Verification items for the finished model (mm, model axes). Face numbers are marked on the shaded views. A direction names the side the tool comes from. Give positions to 0.01 mm unless a question says otherwise; leave off trailing zeros. Order: outer loops, then holes, each group sorted by start corner. A loop starts at its lowest first (then second) coordinate and runs counter-clockwise, first axis right, second up.
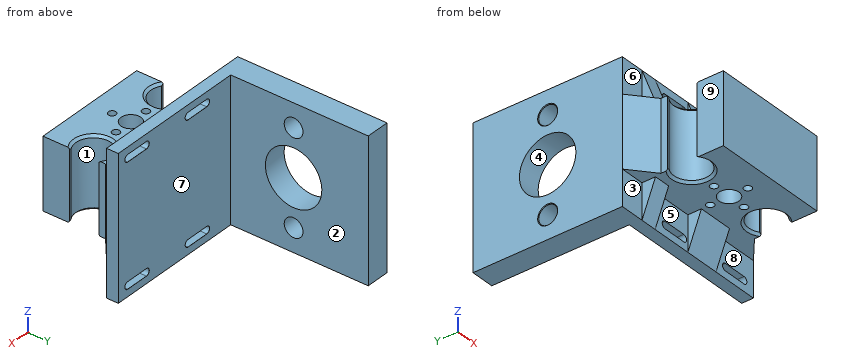
from build123d import *

# Parameters (mm, degrees)
SKETCH_1_W               = 50
SKETCH_1_H               = 35
EXTRUDE_1_DEPTH          = 30
HOLE_WIZARD_362_D        = 8.5
HOLE_WIZARD_467_D        = 3.2
HOLE_WIZARD_621_D        = 15
CHAMFER_1_SIZE           = 1
CHAMFER_1_SIZE_2         = 0.708203932
SKETCH_8_W               = 70
SKETCH_8_H               = 60
SKETCH_8_W_2             = 50
SKETCH_8_H_2             = 30
EXTRUDE_2_DEPTH          = 63.5
HOLE_WIZARD_1_D          = 24
HOLE_WIZARD_2_D          = 8
CHAMFER_2_SIZE           = 0.25
CUT_EXTRUDE_2_DEPTH      = 107.705201373
CUT_EXTRUDE_2_DEPTH_BACK = 107.705201373
SKETCH_14_W              = 60
SKETCH_14_H              = 58.5
MM_START                 = 17
MM_2_DEPTH               = 5.5
RIB_1_REACH              = 95.199
SKETCH_25_WALL_W         = 201.46144539
SKETCH_25_WALL_H         = 30
RIB_2_REACH              = 101.05
SKETCH_26_WALL_W         = 216.17250262
SKETCH_26_WALL_H         = 15
RIB_4_REACH              = 108.5
SKETCH_27_WALL_W         = 231.071518272
SKETCH_27_WALL_H         = 7


with BuildPart() as part:
    # 草图1 → 凸台-拉伸1 (new body)
    with BuildSketch(Plane.XY):
        Rectangle(SKETCH_1_W, SKETCH_1_H)
    extrude(amount=EXTRUDE_1_DEPTH)

    # Hole Wizard 362 (through all)
    with Locations(Plane.XY.offset(30)):
        with Locations((0, 0)):
            Hole(HOLE_WIZARD_362_D / 2)

    # Hole Wizard 467 (through all)
    with Locations(Plane.XY.offset(30)):
        with Locations((8, 0), (0, 8), (-8, 0), (0, -8)):
            Hole(HOLE_WIZARD_467_D / 2)

    # Hole Wizard 621 (through all)
    with Locations(Plane.XY.offset(30)):
        with Locations((20, 0), (-20, 0)):
            Hole(HOLE_WIZARD_621_D / 2)

    # 倒角1
    # the kernel refuses this chamfer: 1, 0.708203932 mm, written as the material it takes off along each edge
    with BuildSketch(Plane(origin=(-20, 0, 0), x_dir=(-0.8790200859122482, 0.4767847402789059, 0), z_dir=(-0.4767847402789059, -0.8790200859122482, 0))) as chamfer_1_piece_1:
        Polygon((7.5, -CHAMFER_1_SIZE), (7.5 + CHAMFER_1_SIZE, 0), (7.5, 0), align=None)
    revolve(axis=Axis((-20, 0, 0), (0, 0, -1)), revolution_arc=303.048763938, mode=Mode.SUBTRACT)
    with BuildSketch(Plane(origin=(-20, 0, 30), x_dir=(-0.879020085912248, 0.47678474027890627, 0), z_dir=(-0.47678474027890627, -0.879020085912248, 0))) as chamfer_1_piece_2:
        Polygon((7.5 + CHAMFER_1_SIZE, 0), (7.5, CHAMFER_1_SIZE), (7.5, 0), align=None)
    revolve(axis=Axis((-20, 0, 30), (0, 0, -1)), revolution_arc=303.048763938, mode=Mode.SUBTRACT)
    with BuildSketch(Plane(origin=(20, 0, 30), x_dir=(0.879020085912248, -0.4767847402789061, 0), z_dir=(0.4767847402789061, 0.879020085912248, 0))) as chamfer_1_piece_3:
        Polygon((7.5 + CHAMFER_1_SIZE, 0), (7.5, CHAMFER_1_SIZE), (7.5, 0), align=None)
    revolve(axis=Axis((20, 0, 30), (0, 0, -1)), revolution_arc=303.048763938, mode=Mode.SUBTRACT)
    with BuildSketch(Plane(origin=(20, 0, 0), x_dir=(0.8790200859122481, 0.476784740278906, 0), z_dir=(0.476784740278906, -0.8790200859122481, 0))) as chamfer_1_piece_4:
        Polygon((7.5, CHAMFER_1_SIZE), (7.5 + CHAMFER_1_SIZE, 0), (7.5, 0), align=None)
    revolve(axis=Axis((20, 0, 0), (0, 0, 1)), revolution_arc=303.048763938, mode=Mode.SUBTRACT)
    with BuildSketch(Plane(origin=(-25, 5.590169944, 32.778051389), x_dir=(0.7914486393779661, 0.611235675682274, 0), z_dir=(0, 0, -1)), Plane(origin=(25, -5.590169944, 32.778051389), x_dir=(-0.7914486393779661, -0.611235675682274, 0), z_dir=(0, 0, -1))) as chamfer_1_piece_5:
        with BuildLine():
            Line((1.080663788, 0), (CHAMFER_1_SIZE_2 * 0.611235676113, -CHAMFER_1_SIZE_2 * 0.791448639936))
            Line((CHAMFER_1_SIZE_2 * 0.611235676113, -CHAMFER_1_SIZE_2 * 0.791448639936), (0, 0))
            ThreePointArc((0, 0), (0.555522087, -0.019473843), (1.080663788, 0))
        make_face()
    extrude(amount=35.556102778, mode=Mode.SUBTRACT)
    with BuildSketch(Plane(origin=(-25, -5.590169944, 32.778051389), x_dir=(0.7914486393779665, -0.6112356756822735, 0), z_dir=(0, 0, -1))) as chamfer_1_piece_6:
        with BuildLine():
            Line((1.080663788, 0), (CHAMFER_1_SIZE_2 * 0.611235676113, CHAMFER_1_SIZE_2 * 0.791448639936))
            Line((CHAMFER_1_SIZE_2 * 0.611235676113, CHAMFER_1_SIZE_2 * 0.791448639936), (0, 0))
            ThreePointArc((0, 0), (0.555522087, 0.019473843), (1.080663788, 0))
        make_face()
    extrude(amount=35.556102778, mode=Mode.SUBTRACT)
    with BuildSketch(Plane(origin=(25, 5.590169944, 32.778051389), x_dir=(0, 1, 0), z_dir=(0, 0, -1))) as chamfer_1_piece_7:
        with BuildLine():
            Line((CHAMFER_1_SIZE_2, 0), (0.660540261, -0.855289885))
            ThreePointArc((0.660540261, -0.855289885), (0.354967464, -0.427764092), (0, 0))
            Line((0, 0), (CHAMFER_1_SIZE_2, 0))
        make_face()
    extrude(amount=35.556102778, mode=Mode.SUBTRACT)

    # 草图8 → 凸台-拉伸2 (add)
    # profile 1 of 5: a face of its own
    with BuildSketch(Plane(origin=(0, 17.5, 0), x_dir=(1, 0, 0), z_dir=(0, 1, 0))):
        with Locations((0, -15)):
            Rectangle(SKETCH_8_W, SKETCH_8_H)
        with Locations((0, -15)):
            Rectangle(SKETCH_8_W_2, SKETCH_8_H_2, mode=Mode.SUBTRACT)
    # profile 2 of 5: a face of its own
    with BuildSketch(Plane(origin=(0, 17.5, 0), x_dir=(1, 0, 0), z_dir=(0, 1, 0))):
        Polygon((25, 0), (0, -15), (25, -30), align=None)
    # profile 3 of 5: a face of its own
    with BuildSketch(Plane(origin=(0, 17.5, 0), x_dir=(1, 0, 0), z_dir=(0, 1, 0))):
        Polygon((25, -30), (0, -15), (-25, -30), align=None)
    # profile 4 of 5: a face of its own
    with BuildSketch(Plane(origin=(0, 17.5, 0), x_dir=(1, 0, 0), z_dir=(0, 1, 0))):
        Polygon((0, -15), (-25, 0), (-25, -30), align=None)
    # profile 5 of 5: a face of its own
    with BuildSketch(Plane(origin=(0, 17.5, 0), x_dir=(1, 0, 0), z_dir=(0, 1, 0))):
        Polygon((25, 0), (-25, 0), (0, -15), align=None)
    extrude(amount=EXTRUDE_2_DEPTH)

    # 孔1 (through all)
    with Locations(Plane(origin=(35, 0, 0), x_dir=(0, 0, -1), z_dir=(1, 0, 0))):
        with Locations((-15, 49.25)):
            Hole(HOLE_WIZARD_1_D / 2)

    # 孔2 (through all)
    with Locations(Plane(origin=(35, 0, 0), x_dir=(0, 0, -1), z_dir=(1, 0, 0))):
        with Locations((5, 49.25), (-35, 49.25)):
            Hole(HOLE_WIZARD_2_D / 2)

    # 倒角2
    chamfer_2_edges = [part.edges().sort_by_distance(p)[0] for p in [
        (-35, 49.25, 31),
        (-35, 49.25, -9),
    ]]
    chamfer(chamfer_2_edges, length=CHAMFER_2_SIZE)

    # 草图14 → 切除-拉伸2 (cut, two sides: drawn at the far end of the back side and taken through both)
    with BuildSketch(Plane.XY.offset(45).offset(-CUT_EXTRUDE_2_DEPTH_BACK)):
        with Locations((5, 51.75)):
            Rectangle(SKETCH_14_W, SKETCH_14_H)
    extrude(amount=CUT_EXTRUDE_2_DEPTH + CUT_EXTRUDE_2_DEPTH_BACK, mode=Mode.SUBTRACT)

    # 大小mm 暗销槽口2: read off the stored shape, not the designer's step
    # 大小mm 暗销槽口2 outline → 大小mm 暗销槽口2 (cut)
    with BuildSketch(Plane(origin=(0, 0, 0), x_dir=(1, 0, 0), z_dir=(0, 1, 0)).offset(MM_START)):
        with BuildLine():
            Line((30, 11.959259259), (20, 11.959259259))
            ThreePointArc((20, 11.959259259), (18.5, 10.459259259), (20, 8.959259259))
            Line((20, 8.959259259), (30, 8.959259259))
            ThreePointArc((30, 8.959259259), (31.5, 10.459259259), (30, 11.959259259))
        make_face()
        with BuildLine():
            ThreePointArc((-12.203065134, 11.959259259), (-13.703065134, 10.459259259), (-12.203065134, 8.959259259))
            Line((-12.203065134, 8.959259259), (-2.203065134, 8.959259259))
            ThreePointArc((-2.203065134, 8.959259259), (-0.703065134, 10.459259259), (-2.203065134, 11.959259259))
            Line((-2.203065134, 11.959259259), (-12.203065134, 11.959259259))
        make_face()
    mm_2 = extrude(amount=MM_2_DEPTH, mode=Mode.SUBTRACT)

    # mm _2 2: loft between two sections, ruled curve by curve
    mm_2_2_from = [
        Edge.make_three_point_arc((30, 22.475, -8.959259259), (31.060660172, 22.475, -9.398599087), (31.5, 22.475, -10.459259259)),
        Edge.make_three_point_arc((31.5, 22.475, -10.459259259), (31.060660172, 22.475, -11.519919431), (30, 22.475, -11.959259259)),
        Edge.make_three_point_arc((20, 22.475, -11.959259259), (18.939339828, 22.475, -11.519919431), (18.5, 22.475, -10.459259259)),
        Edge.make_three_point_arc((18.5, 22.475, -10.459259259), (18.939339828, 22.475, -9.398599087), (20, 22.475, -8.959259259)),
        Edge.make_line((30, 22.475, -11.959259259), (20, 22.475, -11.959259259)),
        Edge.make_line((30, 22.475, -8.959259259), (20, 22.475, -8.959259259)),
    ]
    mm_2_2_to = [
        Edge.make_three_point_arc((30, 22.5, -8.934259259), (31.078337841, 22.5, -9.380921418), (31.525, 22.5, -10.459259259)),
        Edge.make_three_point_arc((31.525, 22.5, -10.459259259), (31.078337841, 22.5, -11.537597101), (30, 22.5, -11.984259259)),
        Edge.make_three_point_arc((20, 22.5, -11.984259259), (18.921662159, 22.5, -11.537597101), (18.475, 22.5, -10.459259259)),
        Edge.make_three_point_arc((18.475, 22.5, -10.459259259), (18.921662159, 22.5, -9.380921418), (20, 22.5, -8.934259259)),
        Edge.make_line((30, 22.5, -11.984259259), (20, 22.5, -11.984259259)),
        Edge.make_line((30, 22.5, -8.934259259), (20, 22.5, -8.934259259)),
    ]
    mm_2_2 = Solid(Shell([*[Face.make_surface_from_curves(mm_2_2_from[k], mm_2_2_to[k]) for k in range(6)], Face(Wire(mm_2_2_from)), Face(Wire(mm_2_2_to))]))
    add(mm_2_2, mode=Mode.SUBTRACT)

    # mm _2 3: loft between two sections, ruled curve by curve
    mm_2_3_from = [
        Edge.make_three_point_arc((-2.203065134, 22.475, -8.959259259), (-1.142404962, 22.475, -9.398599087), (-0.703065134, 22.475, -10.459259259)),
        Edge.make_three_point_arc((-0.703065134, 22.475, -10.459259259), (-1.142404962, 22.475, -11.519919431), (-2.203065134, 22.475, -11.959259259)),
        Edge.make_three_point_arc((-12.203065134, 22.475, -11.959259259), (-13.263725306, 22.475, -11.519919431), (-13.703065134, 22.475, -10.459259259)),
        Edge.make_three_point_arc((-13.703065134, 22.475, -10.459259259), (-13.263725306, 22.475, -9.398599087), (-12.203065134, 22.475, -8.959259259)),
        Edge.make_line((-2.203065134, 22.475, -11.959259259), (-12.203065134, 22.475, -11.959259259)),
        Edge.make_line((-2.203065134, 22.475, -8.959259259), (-12.203065134, 22.475, -8.959259259)),
    ]
    mm_2_3_to = [
        Edge.make_three_point_arc((-2.203065134, 22.5, -8.934259259), (-1.124727293, 22.5, -9.380921418), (-0.678065134, 22.5, -10.459259259)),
        Edge.make_three_point_arc((-0.678065134, 22.5, -10.459259259), (-1.124727293, 22.5, -11.537597101), (-2.203065134, 22.5, -11.984259259)),
        Edge.make_three_point_arc((-12.203065134, 22.5, -11.984259259), (-13.281402975, 22.5, -11.537597101), (-13.728065134, 22.5, -10.459259259)),
        Edge.make_three_point_arc((-13.728065134, 22.5, -10.459259259), (-13.281402975, 22.5, -9.380921418), (-12.203065134, 22.5, -8.934259259)),
        Edge.make_line((-2.203065134, 22.5, -11.984259259), (-12.203065134, 22.5, -11.984259259)),
        Edge.make_line((-2.203065134, 22.5, -8.934259259), (-12.203065134, 22.5, -8.934259259)),
    ]
    mm_2_3 = Solid(Shell([*[Face.make_surface_from_curves(mm_2_3_from[k], mm_2_3_to[k]) for k in range(6)], Face(Wire(mm_2_3_from)), Face(Wire(mm_2_3_to))]))
    add(mm_2_3, mode=Mode.SUBTRACT)

    # 镜向1: 大小mm 暗销槽口2, mm _2 2, mm _2 3 across plane
    add(mm_2.mirror(Plane(origin=(0, 0, 15), x_dir=(1, 0, 0), z_dir=(0, 0, -1))), mode=Mode.SUBTRACT)
    add(mm_2_2.mirror(Plane(origin=(0, 0, 15), x_dir=(1, 0, 0), z_dir=(0, 0, -1))), mode=Mode.SUBTRACT)
    add(mm_2_3.mirror(Plane(origin=(0, 0, 15), x_dir=(1, 0, 0), z_dir=(0, 0, -1))), mode=Mode.SUBTRACT)

    # 草图25 wall → 筋1 (add, up to next)
    with BuildSketch(Plane(origin=(-30, 13.296768148, 15), x_dir=(-0.765461137236, 0.6434821267, 0), z_dir=(0.6434821267, 0.765461137236, 0)), mode=Mode.PRIVATE) as rib_1_sk1:
        Rectangle(SKETCH_25_WALL_W, SKETCH_25_WALL_H)
    rib_1_tool1 = extrude(rib_1_sk1.sketch, amount=RIB_1_REACH, mode=Mode.PRIVATE) - part.part
    rib_1 = rib_1_tool1.solids().sort_by_distance((-30, 13.296768148, 15))[0]
    add(rib_1)

    # 镜向2: 筋1 across plane
    add(rib_1.mirror(Plane(origin=(0, 0, 0), x_dir=(0, 0, 1), z_dir=(1, 0, 0))))

    # 草图26 wall → 筋2 (add, up to next)
    with BuildSketch(Plane(origin=(0, 14.614965359, 37.5), x_dir=(0, 0.359024529342, 0.933328124151), z_dir=(0, -0.933328124151, 0.359024529342)), mode=Mode.PRIVATE) as rib_2_sk1:
        with Locations((0, -7.5)):
            Rectangle(SKETCH_26_WALL_W, SKETCH_26_WALL_H)
    rib_2_tool1 = extrude(rib_2_sk1.sketch, amount=-RIB_2_REACH, mode=Mode.PRIVATE) - part.part
    rib_2 = rib_2_tool1.solids().sort_by_distance((0, 14.614965359, 37.5))[0]
    add(rib_2)

    # 草图27 wall → 筋4 (add, up to next)
    with BuildSketch(Plane(origin=(-17.5, 14.614965359, 37.5), x_dir=(0, -0.359024529342, -0.933328124151), z_dir=(0, 0.933328124151, -0.359024529342)), mode=Mode.PRIVATE) as rib_4_sk1:
        with Locations((0, 3.5)):
            Rectangle(SKETCH_27_WALL_W, SKETCH_27_WALL_H)
    rib_4_tool1 = extrude(rib_4_sk1.sketch, amount=RIB_4_REACH, mode=Mode.PRIVATE) - part.part
    rib_4 = rib_4_tool1.solids().sort_by_distance((-17.5, 14.614965359, 37.5))[0]
    add(rib_4)

    # 镜向4: 筋2, 筋4 across plane
    add(rib_2.mirror(Plane(origin=(0, 0, 15), x_dir=(1, 0, 0), z_dir=(0, 0, -1))))
    add(rib_4.mirror(Plane(origin=(0, 0, 15), x_dir=(1, 0, 0), z_dir=(0, 0, -1))))


solid = part.part
(1) Section check C-C, the plane x = 8. Enter the section's corners in (y, z), then the cut area to 3 significant figures.
Solved:
outline: (-17.5, 0) - (-1.6, 0) - (-1.6, 30) - (-17.5, 30) - close; (1.6, 0) - (11.73, 0) - (17.5, -15) - (22.5, -15) - (22.5, 45) - (17.5, 45) - (11.73, 30) - (1.6, 30) - close
area: 1,340 mm2
(2) Release check for a two-part mould opening along Y. For the marked faces 1, 2, 3 and 4 record: pulls with the +Y half, pulls with the -Y half, needs draft (parallel to the pull), parting line crosses it, or undercut.
Solved:
face 1: undercut
face 2: needs draft
face 3: pulls with the -Y half
face 4: undercut
(3) Go/stop test with flat-tipped pins: pin 1 (4.5 mm diameter, centred on y = 13.5, z = 41, fed in from -X); pin 2 (19.5 mm diameter, centred on x = 20, y = 0, fed in from -Z); pin 3 (1.5 mm diameter, centred on x = 5, z = 30.5, fed in from +Y); pin 4 (3.5 mm diameter, centred on y = -12, z = 16.5, fed in from +X). Record where each tip stops, or that it passes through.
Solved:
pin 1: passes through
pin 2: stops at z = 0
pin 3: stops at y = 22.5
pin 4: stops at x = 25
(4) Section check A-A, the plane z = 15. Enter the section's corners in (x, y).
Solved:
outline: (-35, 17.5) - (-25, 9.09) - (-25, 6.3) - (-24.14, 6.25) arc R7.5 cw (long way) to (-24.14, -6.25) - (-25, -6.3) - (-25, -17.5) - (25, -17.5) - (25, -6.3) - (24.14, -6.25) arc R7.5 cw (long way) to (24.14, 6.25) - (25, 6.3) - (25, 9.09) - (35, 17.5) - (35, 22.5) - (-25, 22.5) - (-25, 37.25) - (-35, 37.25) - close; (-35, 61.25) - (-25, 61.25) - (-25, 81) - (-35, 81) - close; hole circle Ø3.2 at (-8, 0); hole circle Ø8.5 at (0, 0); hole circle Ø3.2 at (0, -8); hole circle Ø3.2 at (0, 8); hole circle Ø3.2 at (8, 0)
(5) Section check B-B, the plane y = 49.25. Enter the section's corners in (x, z).
Solved:
outline: (-35, -15) - (-25, -15) - (-25, -9) - (-34.75, -9) - (-35, -9.25) - close; (-35, -0.75) - (-34.75, -1) - (-25, -1) - (-25, 3) - (-35, 3) - close; (-35, 27) - (-25, 27) - (-25, 31) - (-34.75, 31) - (-35, 30.75) - close; (-35, 39.25) - (-34.75, 39) - (-25, 39) - (-25, 45) - (-35, 45) - close
(6) Scan lines: line 1 (Y direction, x = 0, z = 12.25); line 2 (Z direction, x = 23, y = 20.5); line 3 (Y direction, x = -27.75, z = 35). Record each from-to range of solid material in increasing order.
Solved:
line 1: y = -17.5 to -9.6, -6.4 to -4.25, 4.25 to 6.4, 9.6 to 22.5
line 2: z = -15 to -11.96, -8.96 to 38.96, 41.96 to 45
line 3: y = 17.5 to 45.25, 53.25 to 81
(7) Section check D-D, the plane z = 9. Enter the section's corners in (x, y), then the cut area to 3 significant figures.
Solved:
outline: (-35, 17.5) - (-25, 9.09) - (-25, 6.3) - (-24.14, 6.25) arc R7.5 cw (long way) to (-24.14, -6.25) - (-25, -6.3) - (-25, -17.5) - (25, -17.5) - (25, -6.3) - (24.14, -6.25) arc R7.5 cw (long way) to (24.14, 6.25) - (25, 6.3) - (25, 9.09) - (35, 17.5) - (35, 22.5) - (-25, 22.5) - (-25, 38.86) - (-35, 38.86) - close; (-35, 59.64) - (-25, 59.64) - (-25, 81) - (-35, 81) - close; hole circle Ø3.2 at (-8, 0); hole circle Ø8.5 at (0, 0); hole circle Ø3.2 at (0, -8); hole circle Ø3.2 at (0, 8); hole circle Ø3.2 at (8, 0)
area: 2,160 mm2
(8) Set-up check for the marked faces 5, 6, 7, 8 and 9: record each of +Z, -Z, +X, -X, +Y, -Y from which the full face is reachable in a straight line by a thin tool's end or side.
Solved:
face 5: -Z, -Y
face 6: +Z, -X, -Y
face 7: +Z, -Z, +X, +Y
face 8: -Z, +X, -Y
face 9: +Z, -Z, -X, -Y
